Check sheet for the modelled part. Datum: model origin and axes. Units: mm. Face numbers are marked on the shaded views. A direction names the side the tool comes from. Coordinates: 2 decimals unless noted, no trailing zeros. Loops run counter-clockwise (first coordinate to the right, second up) from the corner with the lowest first, then second, coordinate; pieces in that order, holes last. Notation, with made-up numbers: (-40, -25.5) -> (-13, -25.5) arc R20 ccw to (-13, 4.5) -> close; hole circle Ø8 at (45.25, 74.25). An arc over 180 degrees is marked (long way). Use CSV: the item, a comma, the result in double quotes. Start each with the question number.
1. Release check for a two-part mould opening along X. For the marked faces 1, 2 and 3 record: pulls with the +X half, pulls with the -X half, needs draft (parallel to the pull), parting line crosses it, or undercut.
2. Sectioned sample at C-C, the plane x = 19.82. Record the cut outline in (y, z) (3 decimals), and give its area (3 significant figures).
3. Sectioned sample at A-A, the plane x = -18.5. Record the cut outline in (y, z).
4. Sectioned sample at B-B, the plane z = -1.75. Record the cut outline in (x, y), and give its area (3 significant figures).
5. Sectioned sample at D-D, the plane y = 2.85. Record the cut outline in (x, z) (3 decimals).
6. Set-up check for the marked faces 4 and 5: record each of +Z, -Z, +X, -X, +Y, -Y from which the full face is reachable in a straight line by a thin tool's end or side.
7. Thickness scan on L1, parallel to X at y = 2.15, z = -6; L2, parallel to Z at x = -18.5, y = 3.35; L3, parallel to X at y = 1.3, z = 0 (3 decimals). Record the ranges inside material, lowest first.
8. Gauge pin test, flat end, axial feed: pin 1 (2 mm diameter, centred on x = -7.82, z = 0, fed in from +Y). Record the tip position at first contact, or that the pin passes through.
```python
from build123d import *

# Parameters (mm, degrees)
SKETCH1_W           = 45
SKETCH1_H           = 20
BOSS_EXTRUDE1_DEPTH = 6
SKETCH2_R           = 2.1
CUT_EXTRUDE1_DEPTH  = 6
SKETCH3_R           = 1.175
SKETCH3_W           = 23
SKETCH3_H           = 12.35
CUT_EXTRUDE2_DEPTH  = 6


with BuildPart() as part:
    # Sketch1 → Boss-Extrude1 (new body)
    with BuildSketch(Plane(origin=(0, 0, 0), x_dir=(1, 0, 0), z_dir=(0, 1, 0))):
        Rectangle(SKETCH1_W, SKETCH1_H)
    extrude(amount=BOSS_EXTRUDE1_DEPTH)

    # Sketch2 → Cut-Extrude1 (cut)
    with BuildSketch(Plane(origin=(0, 6, 0), x_dir=(1, 0, 0), z_dir=(0, 1, 0))):
        with Locations((-18.5, -6)):
            Circle(SKETCH2_R)
        with Locations((-18.5, 6)):
            Circle(SKETCH2_R)
    extrude(amount=-CUT_EXTRUDE1_DEPTH, mode=Mode.SUBTRACT)

    # Sketch3 → Cut-Extrude2 (cut)
    with BuildSketch(Plane(origin=(0, 6, 0), x_dir=(1, 0, 0), z_dir=(0, 1, 0))):
        with Locations((-7.82, 0)):
            Circle(SKETCH3_R)
        with Locations((19.82, 0)):
            Circle(SKETCH3_R)
        with Locations((6, 0)):
            Rectangle(SKETCH3_W, SKETCH3_H)
    extrude(amount=-CUT_EXTRUDE2_DEPTH, mode=Mode.SUBTRACT)


solid = part.part
```
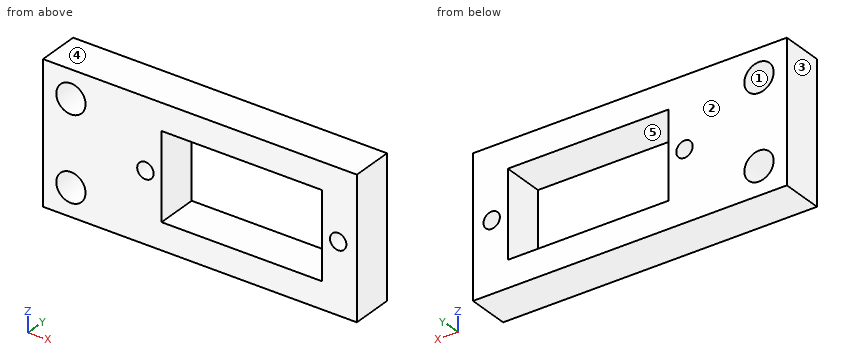
Completed:
1,face 1,"undercut"
1,face 2,"needs draft"
1,face 3,"pulls with the -X half"
2,outline,"(0, -10) -> (6, -10) -> (6, -1.175) -> (0, -1.175) -> close; (0, 1.175) -> (6, 1.175) -> (6, 10) -> (0, 10) -> close"
2,area,"106 mm²"
3,outline,"(0, -10) -> (6, -10) -> (6, -8.1) -> (0, -8.1) -> close; (0, -3.9) -> (6, -3.9) -> (6, 3.9) -> (0, 3.9) -> close; (0, 8.1) -> (6, 8.1) -> (6, 10) -> (0, 10) -> close"
4,outline,"(-22.5, 0) -> (-5.5, 0) -> (-5.5, 6) -> (-22.5, 6) -> close; (17.5, 0) -> (22.5, 0) -> (22.5, 6) -> (17.5, 6) -> close"
4,area,"132 mm²"
5,outline,"(-22.5, -10) -> (22.5, -10) -> (22.5, 10) -> (-22.5, 10) -> close; hole circle Ø4.2 at (-18.5, -6); hole circle Ø4.2 at (-18.5, 6); hole circle Ø2.35 at (-7.82, 0); hole (-5.5, -6.175) -> (17.5, -6.175) -> (17.5, 6.175) -> (-5.5, 6.175) -> close; hole circle Ø2.35 at (19.82, 0)"
6,face 4,"+Z, +X, -X, +Y, -Y"
6,face 5,"+Y, -Y"
7,L1,"-22.5 to -20.6, -16.4 to -5.5, 17.5 to 22.5"
7,L2,"-10 to -8.1, -3.9 to 3.9, 8.1 to 10"
7,L3,"-22.5 to -8.995, -6.645 to -5.5, 17.5 to 18.645, 20.995 to 22.5"
8,pin 1,"through"
